```python
from build123d import *

# Parameters (mm, degrees)
SKETCH2_W           = 126.19
SKETCH2_H           = 25.6
BOSS_EXTRUDE1_DEPTH = 10
SKETCH3_R           = 12.8
SKETCH3_R_2         = 6.55
BOSS_EXTRUDE2_DEPTH = 10
FILLET2_R           = 12.7
CUT_EXTRUDE1_START  = -5.6
SKETCH4_R           = 6.55
CUT_EXTRUDE1_DEPTH  = 5.6


with BuildPart() as part:
    # Sketch2 → Boss-Extrude1 (new body)
    with BuildSketch(Plane.XY):
        Rectangle(SKETCH2_W, SKETCH2_H)
    extrude(amount=BOSS_EXTRUDE1_DEPTH)

    # Sketch3 → Boss-Extrude2 (add)
    with BuildSketch(Plane.XY.offset(10)):
        with Locations(Location((-50.296, 0, 0), (0, 0, 179.283798093))):
            Circle(SKETCH3_R)
        with Locations((-50.296, 0)):
            Circle(SKETCH3_R_2, mode=Mode.SUBTRACT)
    boss_extrude2 = extrude(amount=BOSS_EXTRUDE2_DEPTH)

    # Mirror1: Boss-Extrude2 across plane
    add(boss_extrude2.mirror(Plane(origin=(0, 0, 0), x_dir=(0, 0, 1), z_dir=(1, 0, 0))))

    # Fillet2
    # the kernel refuses this fillet: 12.7 mm, written as the material it takes off along each edge
    with BuildSketch(Plane(origin=(-63.095, -12.8, -31.75), x_dir=(0, 1, 0), z_dir=(0, 0, 1)), Plane(origin=(-63.095, 12.8, -31.75), x_dir=(1, 0, 0), z_dir=(0, 0, 1))) as fillet2_piece_1:
        with BuildLine():
            CenterArc((FILLET2_R, -FILLET2_R), FILLET2_R, 90, 90)
            Line((0, -FILLET2_R), (0, 0))
            Line((0, 0), (FILLET2_R, 0))
        make_face()
    extrude(amount=73.5, mode=Mode.SUBTRACT)
    with BuildSketch(Plane(origin=(63.095, -12.8, -31.75), x_dir=(0, 1, 0), z_dir=(0, 0, 1)), Plane(origin=(63.095, 12.8, -31.75), x_dir=(-1, 0, 0), z_dir=(0, 0, 1))) as fillet2_piece_2:
        with BuildLine():
            CenterArc((FILLET2_R, FILLET2_R), FILLET2_R, 180, 90)
            Line((0, FILLET2_R), (0, 0))
            Line((0, 0), (FILLET2_R, 0))
        make_face()
    extrude(amount=73.5, mode=Mode.SUBTRACT)

    # Sketch4 → Cut-Extrude1 (cut)
    with BuildSketch(Plane.XY.offset(10).offset(CUT_EXTRUDE1_START)):
        with Locations((-50.296, 0)):
            Circle(SKETCH4_R)
    cut_extrude1 = extrude(amount=CUT_EXTRUDE1_DEPTH, mode=Mode.SUBTRACT)

    # Mirror2: Cut-Extrude1 across plane
    add(cut_extrude1.mirror(Plane(origin=(0, 0, 0), x_dir=(0, 0, 1), z_dir=(1, 0, 0))), mode=Mode.SUBTRACT)


solid = part.part
```
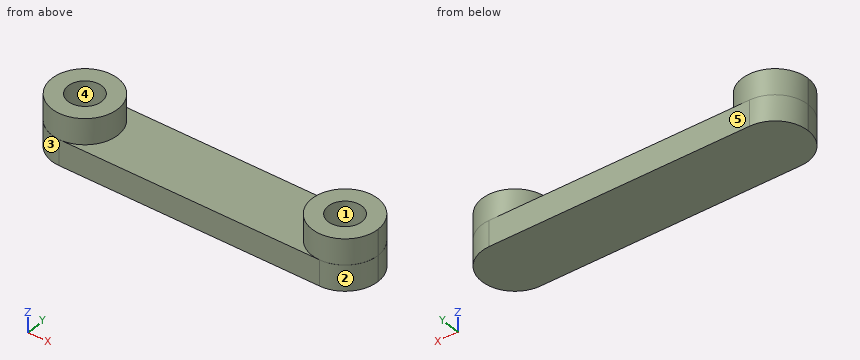
Verification items for the finished model (mm, model axes). Face numbers are marked on the shaded views. A direction names the side the tool comes from. Round coordinates to 2 decimals unless told otherwise and drop trailing zeros. Write each loop counter-clockwise with the first axis right and the second up, starting at its lowest first coordinate (ties: lowest second). Pieces come first, ordered by that corner, then holes.
1. Section check B-B on x = -15.5. Enter the section's corners in (y, z), plus the area to 3 significant figures.
2. Draft check along Y on the marked faces 3, 4 and 5. Enter one of: +Y half, -Y half, draft (parallel to the pull), parting line (faces both ways), or undercut.
3. Section check D-D on y = 9. Enter the section's corners in (x, z).
4. Access from +Z, -Z, +X, -X, +Y, -Y to the whole of each face (thin tool, end or side, straight path). Record for the marked faces 1 and 2.
5. Gauge pin test, flat ends, axial feed: P1, Ø5, axis at y = 4, z = 9.5, coming from the -X side; P2, Ø8, axis at x = -37, y = 4, coming from the -Z side; P3, Ø3, axis at y = -4, z = 9, coming from the -X side. Record the tip position at first contact, or that the pin passes through.
6. Scan lines: L1, parallel to X at y = 1.5, z = 5.75; L2, parallel to X at y = 5.5, z = 13.75; L3, parallel to X at y = -2.5, z = 9.5. Record each from-to range of solid material in increasing order.
Answer:
1. outline: (-12.8, 0) - (12.8, 0) - (12.8, 10) - (-12.8, 10) - close
1. area: 256 mm2
2. face 3: -Y half
2. face 4: undercut
2. face 5: +Y half
3. outline: (-59.45, 0) - (59.45, 0) - (59.45, 10) - (59.4, 10) - (59.4, 20) - (41.19, 20) - (41.19, 10) - (-41.19, 10) - (-41.19, 20) - (-59.4, 20) - (-59.4, 10) - (-59.45, 10) - close
4. face 1: +Z
4. face 2: +Z, -Z, +X, -Y
5. P1: stops at x = -63.02
5. P2: stops at z = 0
5. P3: stops at x = -62.87
6. L1: x = -63.02 to -56.67, -43.92 to 43.92, 56.67 to 63.02
6. L2: x = -61.85 to -53.85, -46.74 to -38.74, 38.74 to 46.74, 53.85 to 61.85
6. L3: x = -62.87 to -56.35, -44.24 to 44.24, 56.35 to 62.87
